Verification items for this drawing (mm, ordinates from the low corner). A direction names the side the tool comes from. Round coordinates to 2 decimals unless told otherwise and drop trailing zeros. Loops run counter-clockwise (first coordinate to the right, second up) from the corner with the lowest first, then second, coordinate; pieces in that order, holes last. Notation, with made-up numbers: M 71,38.5 L 121,38.5 A27 cw 121,71.5 Z; hole C -11.5,-23 d3. An arc over 180 degrees is marked long. Write item = value, one per line.
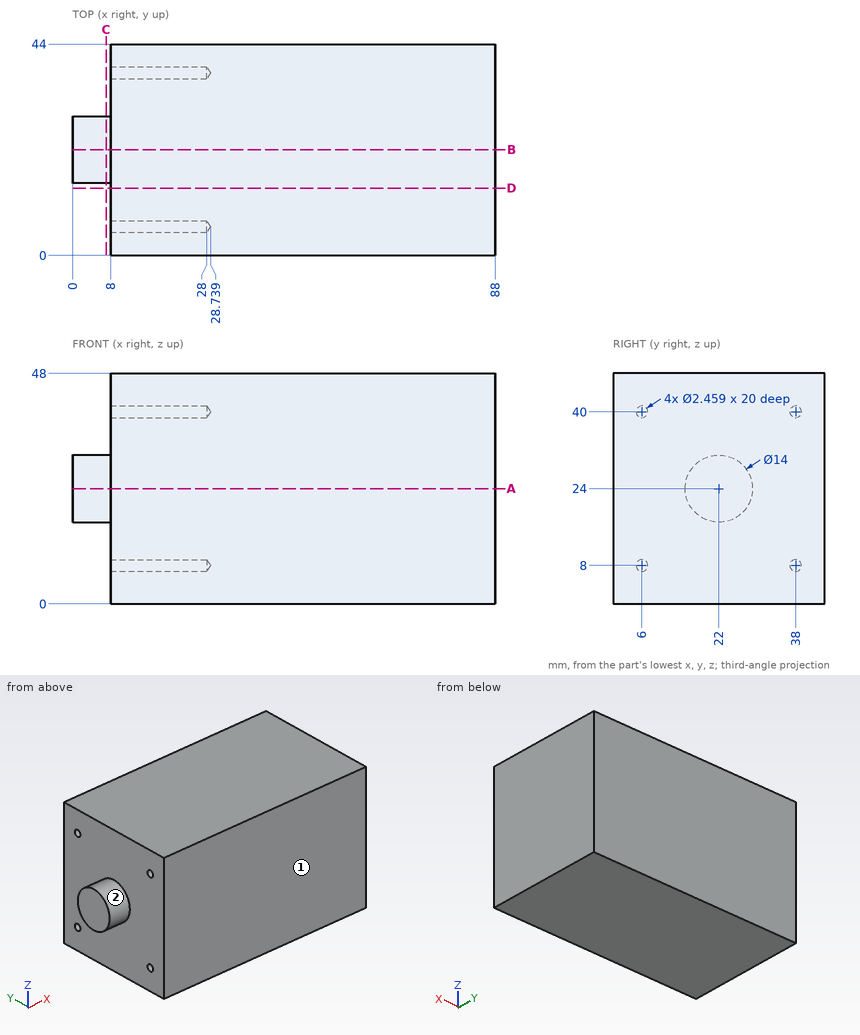
(1) Sectioned sample at C-C on x = 7. Record the cut outline in (y, z), then the cut area to 3 significant figures.
Result set:
outline = C 22,24 d14
area = 154 mm2
(2) Material ranges on line 1 along Y through (x, z) = (12.25, 40); line 2 along Z through (x, y) = (21, 38); line 3 along X through (y, z) = (8.5, 9.5), recorded low to high. Write a range as from..to.
Result set:
line_1 = 0..4.77, 7.23..36.77, 39.23..44
line_2 = 0..6.77, 9.23..38.77, 41.23..48
line_3 = 8..88
(3) Sectioned sample at D-D on y = 14. Record the cut outline in (x, z), then the cut area to 3 significant figures.
Result set:
outline = M 8,0 L 88,0 L 88,48 L 8,48 Z
area = 3,840 mm2
(4) Depth check by flat-ended pin: pin 1 Ø1.5 at (y, z) = (6, 40) entering from -X; pin 2 Ø3 at (y, z) = (6, 8) entering from -X; pin 3 Ø8 at (x, z) = (45.5, 31.5) entering from -Y. Enter the tip coordinate at first touch or a pass-through.
Result set:
pin_1 = 28.29
pin_2 = 8
pin_3 = 0
(5) Sectioned sample at A-A on z = 24. Record the cut outline in (x, y).
Result set:
outline = M 0,15 L 8,15 L 8,0 L 88,0 L 88,44 L 8,44 L 8,29 L 0,29 Z
(6) Sectioned sample at B-B on y = 22. Record the cut outline in (x, z), then the cut area to 3 significant figures.
Result set:
outline = M 0,17 L 8,17 L 8,0 L 88,0 L 88,48 L 8,48 L 8,31 L 0,31 Z
area = 3,950 mm2
(7) Tool access check on the marked faces 1 and 2. Record the directions out of +Z, -Z, +X, -X, +Y, -Y that give a thin tool (end or side, any length) a straight path to the whole face; none if there is none.
Result set:
face_1 = +Z, -Z, +X, -X, -Y
face_2 = -X
